```python
from build123d import *

# Parameters (mm, degrees)
M3_CLEARANCE_HOLE1_D                                = 3.4
SKETCH6_R                                           = 1.7
CUT_EXTRUDE1_DEPTH                                  = 9.5
CUT_EXTRUDE2_REACH                                  = 50.105
SKETCH7_R                                           = 3.25
CBORE_FOR_M3_HEX_SOCKET_HEAD_CAP_SCREW1_D           = 3.4
CBORE_FOR_M3_HEX_SOCKET_HEAD_CAP_SCREW1_CBORE_D     = 6.5
CBORE_FOR_M3_HEX_SOCKET_HEAD_CAP_SCREW1_CBORE_DEPTH = 3.4
CUT_EXTRUDE3_REACH                                  = 70.891
SKETCH12_R                                          = 1.6
CHAMFER1_SIZE                                       = 0.5


with BuildPart() as part:
    # Sketch1 → Revolve1 (revolve)
    with BuildSketch(Plane.XY, mode=Mode.PRIVATE) as revolve1_sk:
        Polygon((0, 32.75), (0, 11), (13, 11), (13, 22.5), (6, 22.5), (6, 24.25), (5.5, 24.25), (5.5, 32.75), align=None)
    revolve(revolve1_sk.sketch.rotate(Axis((0, 0, 0), (1, 0, 0)), 90), axis=Axis((0, 0, 0), (1, 0, 0)))

    # M3 Clearance Hole1 (through all)
    with Locations(Plane(origin=(13, 0, 0), x_dir=(0, 0, -1), z_dir=(1, 0, 0))):
        with Locations((0, 15), (15, 0), (0, -15), (-15, 0)):
            Hole(M3_CLEARANCE_HOLE1_D / 2)

    # Sketch6 → Cut-Extrude1 (cut)
    # profile 1 of 4: a face of its own
    with BuildSketch(Plane.ZY):
        with BuildLine():
            Line((2.75, 10.650704202), (2.75, 16.58771324))
            Line((2.75, 16.58771324), (0, 18.175426481))
            Line((0, 18.175426481), (-2.75, 16.58771324))
            Line((-2.75, 16.58771324), (-2.75, 10.650704202))
            ThreePointArc((-2.75, 10.650704202), (0, 11), (2.75, 10.650704202))
        make_face()
        with Locations(Location((0, 15, 0), (0, 0, 180))):
            Circle(SKETCH6_R, mode=Mode.SUBTRACT)
    # profile 2 of 4: a face of its own
    with BuildSketch(Plane.ZY):
        with BuildLine():
            ThreePointArc((-10.650704202, -2.75), (-11, 0), (-10.650704202, 2.75))
            Line((-10.650704202, 2.75), (-16.58771324, 2.75))
            Line((-16.58771324, 2.75), (-18.175426481, 0))
            Line((-18.175426481, 0), (-16.58771324, -2.75))
            Line((-16.58771324, -2.75), (-10.650704202, -2.75))
        make_face()
        with Locations(Location((-15, 0, 0), (0, 0, 180))):
            Circle(SKETCH6_R, mode=Mode.SUBTRACT)
    # profile 3 of 4: a face of its own
    with BuildSketch(Plane.ZY):
        with BuildLine():
            ThreePointArc((10.650704202, 2.75), (11, 0), (10.650704202, -2.75))
            Line((10.650704202, -2.75), (16.58771324, -2.75))
            Line((16.58771324, -2.75), (18.175426481, 0))
            Line((18.175426481, 0), (16.58771324, 2.75))
            Line((16.58771324, 2.75), (10.650704202, 2.75))
        make_face()
        with Locations(Location((15, 0, 0), (0, 0, 180))):
            Circle(SKETCH6_R, mode=Mode.SUBTRACT)
    # profile 4 of 4: a face of its own
    with BuildSketch(Plane.ZY):
        with BuildLine():
            ThreePointArc((2.75, -10.650704202), (0, -11), (-2.75, -10.650704202))
            Line((-2.75, -10.650704202), (-2.75, -16.58771324))
            Line((-2.75, -16.58771324), (0, -18.175426481))
            Line((0, -18.175426481), (2.75, -16.58771324))
            Line((2.75, -16.58771324), (2.75, -10.650704202))
        make_face()
        with Locations(Location((0, -15, 0), (0, 0, 180))):
            Circle(SKETCH6_R, mode=Mode.SUBTRACT)
    extrude(amount=-CUT_EXTRUDE1_DEPTH, mode=Mode.SUBTRACT)

    # Cut-Extrude2: up to this face of the body (flat: up to its plane)
    cut_extrude2_end = Plane(part.part.faces().sort_by_distance((5.5, 0, -25.176309883))[0])
    # Sketch7 → Cut-Extrude2 (cut, up to the picked face)
    with BuildSketch(Plane(origin=(13, 0, 0), x_dir=(0, 0, -1), z_dir=(1, 0, 0)), mode=Mode.PRIVATE) as cut_extrude2_sk1:
        with Locations((-15.5, 15.5)):
            Circle(SKETCH7_R)
    cut_extrude2_tool1 = split(extrude(cut_extrude2_sk1.sketch, amount=-CUT_EXTRUDE2_REACH, mode=Mode.PRIVATE), bisect_by=cut_extrude2_end, keep=Keep.BOTH, mode=Mode.PRIVATE)
    # Sketch7 → Cut-Extrude2 (cut, up to the picked face)
    with BuildSketch(Plane(origin=(13, 0, 0), x_dir=(0, 0, -1), z_dir=(1, 0, 0)), mode=Mode.PRIVATE) as cut_extrude2_sk2:
        with Locations((-15.5, -15.5)):
            Circle(SKETCH7_R)
    cut_extrude2_tool2 = split(extrude(cut_extrude2_sk2.sketch, amount=-CUT_EXTRUDE2_REACH, mode=Mode.PRIVATE), bisect_by=cut_extrude2_end, keep=Keep.BOTH, mode=Mode.PRIVATE)
    # Sketch7 → Cut-Extrude2 (cut, up to the picked face)
    with BuildSketch(Plane(origin=(13, 0, 0), x_dir=(0, 0, -1), z_dir=(1, 0, 0)), mode=Mode.PRIVATE) as cut_extrude2_sk3:
        with Locations((15.5, -15.5)):
            Circle(SKETCH7_R)
    cut_extrude2_tool3 = split(extrude(cut_extrude2_sk3.sketch, amount=-CUT_EXTRUDE2_REACH, mode=Mode.PRIVATE), bisect_by=cut_extrude2_end, keep=Keep.BOTH, mode=Mode.PRIVATE)
    # Sketch7 → Cut-Extrude2 (cut, up to the picked face)
    with BuildSketch(Plane(origin=(13, 0, 0), x_dir=(0, 0, -1), z_dir=(1, 0, 0)), mode=Mode.PRIVATE) as cut_extrude2_sk4:
        with Locations((15.5, 15.5)):
            Circle(SKETCH7_R)
    cut_extrude2_tool4 = split(extrude(cut_extrude2_sk4.sketch, amount=-CUT_EXTRUDE2_REACH, mode=Mode.PRIVATE), bisect_by=cut_extrude2_end, keep=Keep.BOTH, mode=Mode.PRIVATE)
    add(cut_extrude2_tool1.solids().sort_by(Axis((13, 15.5, 15.5), (-1, 0, 0)))[0], mode=Mode.SUBTRACT)
    add(cut_extrude2_tool2.solids().sort_by(Axis((13, -15.5, 15.5), (-1, 0, 0)))[0], mode=Mode.SUBTRACT)
    add(cut_extrude2_tool3.solids().sort_by(Axis((13, -15.5, -15.5), (-1, 0, 0)))[0], mode=Mode.SUBTRACT)
    add(cut_extrude2_tool4.solids().sort_by(Axis((13, 15.5, -15.5), (-1, 0, 0)))[0], mode=Mode.SUBTRACT)

    # CBORE for M3 Hex Socket Head Cap Screw1 (through all)
    with Locations(Plane(origin=(5.5, 0, 0), x_dir=(0, 0, -1), z_dir=(1, 0, 0))):
        with Locations((-15.5, 15.5), (15.5, 15.5), (15.5, -15.5), (-15.5, -15.5)):
            CounterBoreHole(CBORE_FOR_M3_HEX_SOCKET_HEAD_CAP_SCREW1_D / 2, CBORE_FOR_M3_HEX_SOCKET_HEAD_CAP_SCREW1_CBORE_D / 2, CBORE_FOR_M3_HEX_SOCKET_HEAD_CAP_SCREW1_CBORE_DEPTH)

    # Sketch12 → Cut-Extrude3 (cut, up to next)
    with BuildSketch(Plane(origin=(0, 8.610377228, 20.787289482), x_dir=(-1, 0, 0), z_dir=(0, 0.38268343236508734, 0.9238795325112877)), mode=Mode.PRIVATE) as cut_extrude3_sk1:
        with Locations(Location((-7.8, 0, 0), (0, 0, 90))):
            Circle(SKETCH12_R)
    cut_extrude3_tool1 = extrude(cut_extrude3_sk1.sketch, amount=-CUT_EXTRUDE3_REACH, mode=Mode.PRIVATE) & part.part
    add(cut_extrude3_tool1.solids().sort_by_distance((7.8, 8.610377, 20.787289))[0], mode=Mode.SUBTRACT)

    # Chamfer1
    chamfer1_edges = [part.edges().sort_by_distance(p)[0] for p in [
        (13, 0, -11),
        (13, 22.5, 0),
        (13, 0, -22.5),
        (13, -22.5, 0),
        (13, 0, 22.5),
        (13, -13.201902961, 13.201902961),
        (13, -13.201902961, -13.201902961),
        (13, 13.201902961, -13.201902961),
        (13, 13.201902961, 13.201902961),
        (13, 15, -1.7),
        (13, 0, 13.3),
        (13, -15, -1.7),
        (13, 0, -16.7),
        (0, 7.778174593, -7.778174593),
        (0, -7.778174593, -7.778174593),
        (0, -7.778174593, 7.778174593),
        (0, 13.619208721, -2.75),
        (0, 13.619208721, 2.75),
        (0, 17.38156986, 1.375),
        (0, 17.38156986, -1.375),
        (0, 2.75, 13.619208721),
        (0, -2.75, 13.619208721),
        (0, -1.375, 17.38156986),
        (0, 1.375, 17.38156986),
        (0, 7.778174593, 7.778174593),
        (0, -13.619208721, -2.75),
        (0, -17.38156986, -1.375),
        (0, -17.38156986, 1.375),
        (0, -13.619208721, 2.75),
        (0, 0, -32.75),
        (5.5, 0, -32.75),
        (0, 2.75, -13.619208721),
        (0, 1.375, -17.38156986),
        (0, -1.375, -17.38156986),
        (0, -2.75, -13.619208721),
    ]]
    chamfer(chamfer1_edges, length=CHAMFER1_SIZE)


solid = part.part
```
Geometry check sheet. Reference: the model listing, model coordinates, mm. A direction names the side the tool comes from. Coordinates: 2 decimals unless noted, no trailing zeros. Loops run counter-clockwise (first coordinate to the right, second up) from the corner with the lowest first, then second, coordinate; pieces in that order, holes last.
Item 1: Sectioned sample at A-A, the plane x = 4. Record the boundary of the cut face in (y, z).
Item 2: Release check for a two-part mould opening along Y. For faces 4 (the face through (12.64, -13.05, -13.16)), 5 (the face through (1.04, -16.15, 17.07)), 6 (the face through (13, 9, -9)), 7 (the face through (9.2, -22.5, 0.2)) record: released by +Y, released by -Y, zero draft, split by the parting line, or undercut.
Item 3: Thickness scan on line 1 (Y direction, x = 11.75, z = 0); line 2 (Y direction, x = 1, z = 15.5); line 3 (X direction, y = 23, z = 17.5). Record the ranges inside material, lowest first.
Item 4: Access from +Z, -Z, +X, -X, +Y, -Y to the whole of each face (thin tool, end or side, straight path). Record for faces 1 (the face through (5.5, -24, -5)), 2 (the face through (0.365, 7.815, -7.932)), 3 (the face through (9.2, 0.2, 22.5)).
Item 5: Go/stop test with flat-tipped pins: pin 1 Ø4.5 at (x, y) = (4.5, -15) entering from -Z; pin 2 Ø2 at (y, z) = (-15, -16.5) entering from +X; pin 3 Ø5 at (x, y) = (4, -21) entering from -Z. Record where each tip stops, or that it passes through.
Check result:
1. outline: circle Ø65.5 at (0, 0); hole circle Ø6.5 at (-15.5, -15.5); hole circle Ø6.5 at (-15.5, 15.5); hole (-18.18, 0) - (-16.59, -2.75) - (-10.65, -2.75) arc R11 ccw to (-2.75, -10.65) - (-2.75, -16.59) - (0, -18.18) - (2.75, -16.59) - (2.75, -10.65) arc R11 ccw to (10.65, -2.75) - (16.59, -2.75) - (18.18, 0) - (16.59, 2.75) - (10.65, 2.75) arc R11 ccw to (2.75, 10.65) - (2.75, 16.59) - (0, 18.18) - (-2.75, 16.59) - (-2.75, 10.65) arc R11 ccw to (-10.65, 2.75) - (-16.59, 2.75) - close; hole circle Ø6.5 at (15.5, -15.5); hole circle Ø6.5 at (15.5, 15.5)
2. face 4: undercut
2. face 5: undercut
2. face 6: zero draft
2. face 7: released by -Y
3. line 1: y = -22.5 to -16.7, -13.3 to -11, 11 to 13.3, 16.7 to 22.5
3. line 2: y = -28.85 to -17.2, -13.8 to -2.75, 2.75 to 13.8, 17.2 to 28.85
3. line 3: x = 0 to 5.5
4. face 1: +X
4. face 2: -X
4. face 3: +Z, +X
5. pin 1: stops at z = -30.17
5. pin 2: stops at x = 2.1
5. pin 3: stops at z = -27.02
